from build123d import *

# Parameters (mm, degrees)
F0_W     = 89
F0_H     = 37
F0_R     = 1.5
F1_DEPTH = 1.5
F2_W     = 12.5
F2_H     = 12
F2_W_2   = 3.5
F3_DEPTH = 11.5
F2_W_3   = 7
F2_H_2   = 20.3
F2_W_4   = 2
F4_DEPTH = 9


with BuildPart() as f1:
    # F0 (on Top) → F1 (new body)
    with BuildSketch(Plane.XY):
        Rectangle(F0_W, F0_H)
        with Locations((-40, -15)):
            Circle(F0_R, mode=Mode.SUBTRACT)
        with Locations((-10, -1)):
            Circle(F0_R, mode=Mode.SUBTRACT)
        with Locations((40, -15)):
            Circle(F0_R, mode=Mode.SUBTRACT)
        with Locations((-40, 15)):
            Circle(F0_R, mode=Mode.SUBTRACT)
        with Locations((40, 15)):
            Circle(F0_R, mode=Mode.SUBTRACT)
    extrude(amount=F1_DEPTH)

    # F2 (on face) → F3 (join)
    with BuildSketch(Plane(origin=(0, 0, 0), x_dir=(1, 0, 0), z_dir=(0, 0, -1))):
        with Locations((-38.25, 0)):
            Rectangle(F2_W, F2_H)
        with Locations((-46.25, 0)):
            Rectangle(F2_W_2, F2_H)
    extrude(amount=F3_DEPTH)

    # F2 (on face) → F4 (join)
    with BuildSketch(Plane(origin=(0, 0, 0), x_dir=(1, 0, 0), z_dir=(0, 0, -1))):
        with Locations((48, 0)):
            Rectangle(F2_W_3, F2_H_2)
        with Locations((43.5, 0)):
            Rectangle(F2_W_4, F2_H_2)
    extrude(amount=F4_DEPTH)


solid = f1.part
Verification items for the finished model (mm, model axes). A direction names the side the tool comes from. Coordinates: 2 decimals unless noted, no trailing zeros. Loops run counter-clockwise (first coordinate to the right, second up) from the corner with the lowest first, then second, coordinate; pieces in that order, holes last. Notation, with made-up numbers: (45, -24) -> (82, -24) arc R23 ccw to (82, -13) -> close; hole circle Ø3 at (30, 16). An arc over 180 degrees is marked (long way). Answer as a JSON object with one key per item and string values. Group by question number.
Item 1: Mould release check, pull along Y, two halves, no side actions. Record for faces 1 (the cylindrical face through (-41.5, -14.93, 0.74)), 2 (the flat face through (47, 10.15, -4)), 3 (the flat face through (-46, 0, 0)): +Y half, -Y half, draft (parallel to the pull), parting line (faces both ways), or undercut.
Item 2: Depth check by flat-ended pin: pin 1 (3 mm diameter, centred on x = -46.5, y = 3, fed in from +Z); pin 2 (5 mm diameter, centred on x = -24.5, y = -7, fed in from -Z); pin 3 (6 mm diameter, centred on y = 11, z = -4.5, fed in from -X). Enter the tip coordinate at first touch or a pass-through.
Item 3: Sectioned sample at B-B on z = -2.25. Record the boundary of the cut face in (x, y).
Item 4: Sectioned sample at D-D on y = 15. Record the boundary of the cut face in (x, z).
Item 5: Sectioned sample at C-C on x = -10. Record the boundary of the cut face in (y, z).
Item 6: Sectioned sample at A-A on y = -1. Record the boundary of the cut face in (x, z).
Item 7: Tool access check on faces 4 (the flat face through (-40, -6, -6)), 5 (the flat face through (47, 0, -9)), 6 (the flat face through (48, 0, 0)), 7 (the flat face through (47, -10.15, -4)), 8 (the flat face through (42.5, 0, -4)). Record the directions out of +Z, -Z, +X, -X, +Y, -Y that give a thin tool (end or side, any length) a straight path to the whole face; none if there is none.
Item 8: Scan lines: probe 1 along Y at (x, z) = (-40, 1.15); probe 2 along Z at (x, y) = (27, 6); probe 3 along X at (y, z) = (1, -10.25). Record each from-to range of solid material in increasing order.
Evaluation:
{
 "1": {"face 1": "undercut", "face 2": "+Y half", "face 3": "draft"},
 "2": {"pin 1": "stops at z = 0", "pin 2": "stops at z = 0", "pin 3": "stops at x = 42.5"},
 "3": {"outline": "(-48, -6) -> (-32, -6) -> (-32, 6) -> (-48, 6) -> close; (42.5, -10.15) -> (51.5, -10.15) -> (51.5, 10.15) -> (42.5, 10.15) -> close"},
 "4": {"outline": "(-44.5, 0) -> (-41.5, 0) -> (-41.5, 1.5) -> (-44.5, 1.5) -> close; (-38.5, 0) -> (38.5, 0) -> (38.5, 1.5) -> (-38.5, 1.5) -> close; (41.5, 0) -> (44.5, 0) -> (44.5, 1.5) -> (41.5, 1.5) -> close"},
 "5": {"outline": "(-18.5, 0) -> (-2.5, 0) -> (-2.5, 1.5) -> (-18.5, 1.5) -> close; (0.5, 0) -> (18.5, 0) -> (18.5, 1.5) -> (0.5, 1.5) -> close"},
 "6": {"outline": "(-48, -11.5) -> (-32, -11.5) -> (-32, 0) -> (-11.5, 0) -> (-11.5, 1.5) -> (-44.5, 1.5) -> (-44.5, 0) -> (-48, 0) -> close; (-8.5, 0) -> (42.5, 0) -> (42.5, -9) -> (51.5, -9) -> (51.5, 0) -> (44.5, 0) -> (44.5, 1.5) -> (-8.5, 1.5) -> close"},
 "7": {"face 4": "-Z, -X, -Y", "face 5": "-Z, +X, +Y, -Y", "face 6": "+Z, +X, +Y, -Y", "face 7": "-Z, +X, -X, -Y", "face 8": "-Z, +Y, -Y"},
 "8": {"probe 1": "y = -18.5 to -16.5, -13.5 to 13.5, 16.5 to 18.5", "probe 2": "z = 0 to 1.5", "probe 3": "x = -48 to -32"}
}
